For this review, take the finished solid that the model builds, in its own axes (mm). Face numbers are marked on the shaded views. Give positions to 0.01 mm unless a question says otherwise; leave off trailing zeros. Write each loop counter-clockwise with the first axis right and the second up, starting at its lowest first coordinate (ties: lowest second). Pieces come first, ordered by that corner, then holes.
Autodesk Inventor part; units mm, degrees
ref_plane "YZ Plane" through (0, 0, 0) normal (1, 0, 0) x (0, 1, 0)
ref_plane "XZ Plane" through (0, 0, 0) normal (0, 1, 0) x (-1, 0, 0)
ref_plane "XY Plane" through (0, 0, 0) normal (0, 0, 1) x (1, 0, 0)
sketch "Sketch1" plane through (0, 0, 0) normal (0, 0, 1) x (1, 0, 0)
  line L0 (0, 0) -> (0, 42.85)
  line L1 (52.35, 95.2) -> (69.8, 95.2)
  arc A0 (52.35, 95.2) -> (0, 42.85) centre (52.35, 42.85) ccw
  dimension "d1" = 95.2
  dimension "d2" = 69.8
  dimension "d4" = 52.35
sketch "Sketch2" plane through (0, 0, 0) normal (0, 1, 0) x (-1, 0, 0)
  circle A0 centre (0, 0) radius 19.05
  circle A1 centre (0, 0) radius 17.4
  dimension "d3" = 38.1
  dimension "d11" = 1.65
sweep "Sweep1" add profiles "Sketch2" path "Sketch1"
sketch "Sketch3" plane through (69.8, 95.2, 0) normal (1, 0, 0) x (0, 0, -1)
  circle A0 centre (0, 0) radius 19.05
  circle A1 centre (0, 0) radius 25.15
  point P0 (0, -95.2)
  dimension "d6" = 50.3
extrude "Extrusion1" add sketch "Sketch3" against normal blind 5
chamfer "Chamfer1" distance 3 distance2 3.8692 1 edges at (64.8, 95.2, 25.15) measured on face at (66.4667, 91.1657, -24.8243)
equation "\"d4\" = 0.75 * d2"
equation "\"d15\" = 0.0769231 * d6"
properties part number "Ferrule 90 deg Elb-38.1"
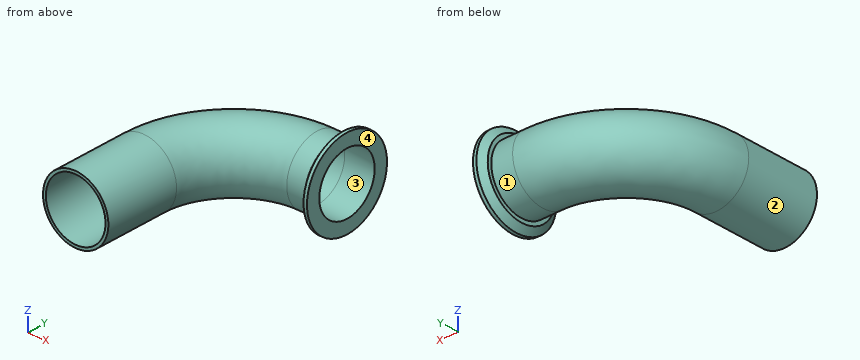
(1) For L1, parallel to Y at x = 57, z = 0; L2, parallel to X at y = 70, z = -10.5; L3, parallel to Y at x = 48, z = 1, list the stretches that pass through material, from the lowest coordinate up.
(2) We need section B-B (y = 36). Write out the cut boundary in (x, z).
(3) Clearance check with flat-ended pins moving along their axes: pin 1 Ø10 at (x, z) = (47, 0.5) entering from +Y; pin 2 Ø12 at (x, y) = (-9, 48.5) entering from +Z; pin 3 Ø12 at (x, z) = (43, 19) entering from -Y. State where each tip first meets the part, or that it passes through.
(4) We need section A-A (z = 0). Write out the cut boundary in (x, y).
(5) The part is to be moulded in two halves that separate along X. For the marked faces 1, 2, 3 and 4, say which applies: +X half, -X half, draft (parallel to the pull), parting line (faces both ways), or undercut.
The answers:
1. L1: y = 76.15 to 77.8, 112.6 to 114.25
1. L2: x = -10.26 to -8.05, 25.09 to 28.02
1. L3: y = 75.89 to 77.56, 112.44 to 114.09
2. outline: circle Ø38.1 at (0, 0); hole circle Ø34.8 at (0, 0)
3. pin 1: stops at y = 114.25
3. pin 2: stops at z = 18.77
3. pin 3: stops at y = 79.9
4. outline: (-19.05, 0) - (-17.4, 0) - (-17.4, 42.85) arc R69.75 cw to (52.35, 112.6) - (69.8, 112.6) - (69.8, 120.35) - (67.8, 120.35) - (64.8, 116.48) - (64.8, 114.25) - (52.35, 114.25) arc R71.4 ccw to (-19.05, 42.85) - close; (17.4, 0) - (19.05, 0) - (19.05, 42.85) arc R33.3 cw to (52.35, 76.15) - (64.8, 76.15) - (64.8, 73.92) - (67.8, 70.05) - (69.8, 70.05) - (69.8, 77.8) - (52.35, 77.8) arc R34.95 ccw to (17.4, 42.85) - close
5. face 1: undercut
5. face 2: parting line
5. face 3: draft
5. face 4: +X half
